from build123d import *

# Parameters (mm, degrees)
SKETCH1_W                                      = 24
SKETCH1_H                                      = 18
SKETCH1_W_2                                    = 3.25
SKETCH1_H_2                                    = 3.25
BOSS_EXTRUDE1_DEPTH                            = 20
FILLET1_R                                      = 3
SKETCH2_W                                      = 6.1
SKETCH2_H                                      = 6.1
CUT_EXTRUDE1_DEPTH                             = 3
SKETCH3_W                                      = 9.25
SKETCH3_H                                      = 8.1
CUT_EXTRUDE2_DEPTH                             = 28.730849248
SKETCH4_W                                      = 3.25
SKETCH4_H                                      = 3.25
BOSS_EXTRUDE2_DEPTH                            = 2.95
CBORE_FOR_6_SOCKET_HEAD_CAP_SCREW1_D           = 3.6576
CBORE_FOR_6_SOCKET_HEAD_CAP_SCREW1_CBORE_D     = 7.14502
CBORE_FOR_6_SOCKET_HEAD_CAP_SCREW1_CBORE_DEPTH = 3.5052


with BuildPart() as part:
    # Sketch1 → Boss-Extrude1 (new body)
    # profile 1 of 2: a face of its own
    with BuildSketch(Plane.XY):
        Rectangle(SKETCH1_W, SKETCH1_H)
        Rectangle(SKETCH1_W_2, SKETCH1_H_2, mode=Mode.SUBTRACT)
    # profile 2 of 2: a face of its own
    with BuildSketch(Plane.XY):
        Polygon((-1.625, -1.625), (-1.625, 1.625), (-1.625, 4), (-4.8, 4), (-4.8, -4), (-1.625, -4), align=None)
    extrude(amount=BOSS_EXTRUDE1_DEPTH)

    # Fillet1
    fillet1_edges = [part.edges().sort_by_distance(p)[0] for p in [
        (12, 0, 0),
        (0, -9, 0),
        (-12, -9, 10),
        (-12, 9, 10),
        (12, 9, 10),
        (12, -9, 10),
        (-12, 0, 0),
        (0, 9, 0),
    ]]
    fillet(fillet1_edges, radius=FILLET1_R)

    # Sketch2 → Cut-Extrude1 (cut)
    with BuildSketch(Plane(origin=(0, 9, 0), x_dir=(1, 0, 0), z_dir=(0, 1, 0))):
        with Locations((-5, -8)):
            Rectangle(SKETCH2_W, SKETCH2_H)
        with Locations((5, -8)):
            Rectangle(SKETCH2_W, SKETCH2_H)
    extrude(amount=-CUT_EXTRUDE1_DEPTH, mode=Mode.SUBTRACT)

    # Sketch3 → Cut-Extrude2 (cut, through all)
    with BuildSketch(Plane(origin=(0, 6, 0), x_dir=(1, 0, 0), z_dir=(0, 1, 0))):
        with Locations((0, -7)):
            Rectangle(SKETCH3_W, SKETCH3_H)
    extrude(amount=-CUT_EXTRUDE2_DEPTH, mode=Mode.SUBTRACT)

    # Sketch4 → Boss-Extrude2 (add)
    with BuildSketch(Plane(origin=(0, 0, 0), x_dir=(-1, 0, 0), z_dir=(0, 0, -1))):
        Rectangle(SKETCH4_W, SKETCH4_H)
    extrude(amount=-BOSS_EXTRUDE2_DEPTH)

    # CBORE for #6 Socket Head Cap Screw1 (through all)
    with Locations(Plane(origin=(12, 0, 0), x_dir=(0, 0, -1), z_dir=(1, 0, 0))):
        with Locations((-7.025, 0)):
            CounterBoreHole(CBORE_FOR_6_SOCKET_HEAD_CAP_SCREW1_D / 2, CBORE_FOR_6_SOCKET_HEAD_CAP_SCREW1_CBORE_D / 2, CBORE_FOR_6_SOCKET_HEAD_CAP_SCREW1_CBORE_DEPTH)


solid = part.part
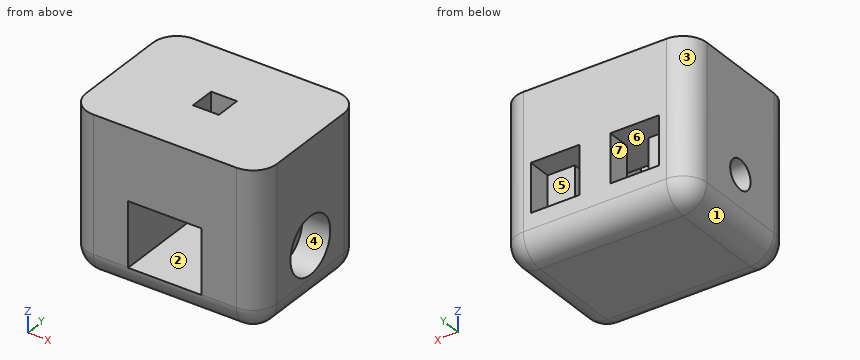
The listing builds one solid part. Answer for the finished solid, in the listing's coordinates (mm). Face numbers are marked on the shaded views. A direction names the side the tool comes from. Give positions to 0.01 mm unless a question says otherwise; leave off trailing zeros. Write each loop counter-clockwise with the first axis right and the second up, starting at its lowest first coordinate (ties: lowest second). Pieces come first, ordered by that corner, then holes. Notation, with made-up numbers: (-23, 17.5) -> (22, 17.5) arc R22 ccw to (22, 48.5) -> close; hole circle Ø4 at (-31, -29.75). An arc over 180 degrees is marked (long way). Use a Markdown table: item, result.
(1) Section C-C, the plane x = -2.5 is taken. Determine the outline of the cut face in (y, z).
Return value:
| item | result |
|---|---|
| outline | (-9, 2.95) arc R3 ccw to (-6, 0) -> (6, 0) arc R3 ccw to (9, 3) -> (9, 4.95) -> (6, 4.95) -> (6, 2.95) -> close; (-9, 11.05) -> (9, 11.05) -> (9, 20) -> (-9, 20) -> close |
(2) Section A-A, the plane z = 13 is taken. Determine the outline of the cut face in (x, y) (3 decimals).
Return value:
| item | result |
|---|---|
| outline | (-12, -6) arc R3 ccw to (-9, -9) -> (9, -9) arc R3 ccw to (12, -6) -> (12, 6) arc R3 ccw to (9, 9) -> (-9, 9) arc R3 ccw to (-12, 6) -> close; hole (-1.625, -1.625) -> (1.625, -1.625) -> (1.625, 1.625) -> (-1.625, 1.625) -> close |
(3) Section B-B, the plane y = 4.5 is taken. Determine the outline of the cut face in (x, z) (3 decimals).
Return value:
| item | result |
|---|---|
| outline | (-12, 3) arc R3 ccw to (-9, 0) -> (9, 0) arc R3 ccw to (12, 3) -> (12, 20) -> (-12, 20) -> close; hole (-4.625, 2.95) -> (4.625, 2.95) -> (4.625, 11.05) -> (-4.625, 11.05) -> close |
(4) Section D-D, the plane y = 0 is taken. Give the number of separate pieces and of enclosed holes in the cut face, then the cut area to 3 significant figures.
Return value:
| item | result |
|---|---|
| separate pieces | 3 |
| enclosed holes | 0 |
| area | 306 mm2 |
(5) Determine the mould class of the marked faces 1, 2 and 3 for opening direction Z: released by +Z, released by -Z, zero draft, split by the parting line, or undercut.
Return value:
| item | result |
|---|---|
| face 1 | released by -Z |
| face 2 | undercut |
| face 3 | zero draft |
(6) Flat-ended cylindrical pins translate along their axes: P1, Ø1.5, axis at y = 7.5, z = 8.5, coming from the +X side; P2, Ø8, axis at y = 0, z = 7.025, coming from the -X side; P3, Ø6, axis at y = 0, z = 7.025, coming from the +X side; P4, Ø0.9, axis at y = 7.5, z = 8.5, coming from the -X side. Find the tip coordinate at first contact, or state that the pin passes through.
Return value:
| item | result |
|---|---|
| P1 | x = 11.9 |
| P2 | x = -12 |
| P3 | x = 8.49 |
| P4 | x = -11.81 |
(7) For the marked faces 4, 5, 6 and 7, determine the directions among +Z, -Z, +X, -X, +Y, -Y from which every point of the face is accessible in a straight line to the end or side of a thin tool.
Return value:
| item | result |
|---|---|
| face 4 | +X |
| face 5 | +Y |
| face 6 | none |
| face 7 | +Y, -Y |
(8) Find the intervals of material crossed by probe 1 along X at (y, z) = (-2.5, 8) (3 decimals); probe 2 along X at (y, z) = (3.5, 4) (3 decimals); probe 3 along Y at (x, z) = (1.75, 9), in increasing order. Write a range as from..to.
Return value:
| item | result |
|---|---|
| probe 1 | -12..-4.625, 4.625..8.495 |
| probe 2 | -12..-4.625, 4.625..12 |
| probe 3 | 6..9 |
